Check sheet for the modelled part. Datum: model origin and axes. Units: mm. A direction names the side the tool comes from. Coordinates: 2 decimals unless noted, no trailing zeros. Loops run counter-clockwise (first coordinate to the right, second up) from the corner with the lowest first, then second, coordinate; pieces in that order, holes last. Notation, with made-up numbers: (15, -20.5) -> (37, -20.5) arc R16 ccw to (37, -12.5) -> close; hole circle Ø9 at (74.5, 29). An arc over 180 degrees is marked (long way). Use CSV: the item, a comma, the result in double quotes.
```python
from build123d import *

# Parameters (mm, degrees)
SKETCH_R           = 10.3
PAD_DEPTH          = 2
SKETCH001_R        = 4.3
SKETCH001_R_2      = 3.3
POCKET_DEPTH       = 1
SKETCH002_R        = 2.8
POCKET001_DEPTH    = 1
SKETCH003_R        = 1.5
POCKET002_DEPTH    = 1.001
SKETCH004_R        = 4.5
SKETCH004_R_2      = 3
PAD001_DEPTH       = 3
SKETCH005_R        = 0.75
POCKET003_DEPTH    = 5
POLARPATTERN_COUNT = 4


with BuildPart() as part:
    # Sketch → Pad (new body)
    with BuildSketch(Plane.XY):
        Circle(SKETCH_R)
    extrude(amount=PAD_DEPTH)

    # Sketch001 (on Face2 of Pad) → Pocket (cut)
    with BuildSketch(Plane(origin=(0, 0, 0), x_dir=(1, 0, 0), z_dir=(0, 0, -1))):
        Circle(SKETCH001_R)
        Circle(SKETCH001_R_2, mode=Mode.SUBTRACT)
    extrude(amount=-POCKET_DEPTH, mode=Mode.SUBTRACT)

    # Sketch002 (on Face7 of Pocket) → Pocket001 (cut)
    with BuildSketch(Plane(origin=(0, 0, 0), x_dir=(1, 0, 0), z_dir=(0, 0, -1))):
        Circle(SKETCH002_R)
    extrude(amount=-POCKET001_DEPTH, mode=Mode.SUBTRACT)

    # Sketch003 (on Face9 of Pocket001) → Pocket002 (cut, through all)
    with BuildSketch(Plane(origin=(0, 0, 1), x_dir=(1, 0, 0), z_dir=(0, 0, -1))):
        Circle(SKETCH003_R)
    extrude(amount=-POCKET002_DEPTH, mode=Mode.SUBTRACT)

    # Sketch004 (on Face3 of Pocket002) → Pad001 (join)
    with BuildSketch(Plane.XY.offset(2)):
        Circle(SKETCH004_R)
        Circle(SKETCH004_R_2, mode=Mode.SUBTRACT)
    extrude(amount=PAD001_DEPTH)

    # Sketch005 (on Face2 of Pad001) → Pocket003 (cut)
    with BuildSketch(Plane(origin=(0, 0, 0), x_dir=(1, 0, 0), z_dir=(0, 0, -1))):
        with Locations((-3.3, 7.3)):
            Circle(SKETCH005_R)
        with Locations((0, 7.3)):
            Circle(SKETCH005_R)
        with Locations((3.3, 7.3)):
            Circle(SKETCH005_R)
    pocket003 = extrude(amount=-POCKET003_DEPTH, mode=Mode.SUBTRACT)

    # PolarPattern: Pocket003 ×4 about axis
    polarpattern_axis = Axis((0, 0, 0), (0, 0, -1))
    for i in range(1, POLARPATTERN_COUNT):
        add(pocket003.rotate(polarpattern_axis, i * 360 / POLARPATTERN_COUNT), mode=Mode.SUBTRACT)


solid = part.part
```
1) Go/stop test with flat-tipped pins: pin 1 Ø2.5 at (x, y) = (0, 0) entering from -Z; pin 2 Ø2 at (x, y) = (3.3, 7.3) entering from -Z; pin 3 Ø1.7 at (x, y) = (7.3, -3.3) entering from +Z. Record where each tip stops, or that it passes through.
Answer below:
pin 1,"passes through"
pin 2,"stops at z = 0"
pin 3,"stops at z = 2"
2) Cross-section at A-A on x = -3.75. Record the boundary of the cut face in (y, z).
Answer below:
outline,"(-9.59, 0) -> (-7.9, 0) -> (-7.9, 2) -> (-9.59, 2) -> close; (-6.7, 0) -> (-2.1, 0) -> (-2.1, 1) -> (2.1, 1) -> (2.1, 0) -> (6.7, 0) -> (6.7, 2) -> (2.49, 2) -> (2.49, 5) -> (-2.49, 5) -> (-2.49, 2) -> (-6.7, 2) -> close; (7.9, 0) -> (9.59, 0) -> (9.59, 2) -> (7.9, 2) -> close"
3) Thickness scan on line 1 along Y through (x, z) = (0, 0.35); line 2 along Y through (x, z) = (0, 1.3); line 3 along Y through (x, z) = (0, 2.9). Record the ranges inside material, lowest first. Write a range as from..to.
Answer below:
line 1,"y = -10.3..-8.05, -6.55..-4.3, -3.3..-2.8, 2.8..3.3, 4.3..6.55, 8.05..10.3"
line 2,"y = -10.3..-8.05, -6.55..-1.5, 1.5..6.55, 8.05..10.3"
line 3,"y = -4.5..-3, 3..4.5"
4) Draft check along X on faces 4 (the cylindrical face through (9.824, 3.094, 0.986)), 5 (the flat face through (2.1, -4.4, 2)), 6 (the cylindrical face through (-3.202, 8.044, 0.986)), 7 (the cylindrical face through (-3, 0, 3)). Enter one of: released by +X, released by -X, zero draft, split by the parting line, or undercut.
Answer below:
face 4,"split by the parting line"
face 5,"zero draft"
face 6,"undercut"
face 7,"undercut"
5) Cross-section at B-B on x = 7.3. Record the boundary of the cut face in (y, z).
Answer below:
outline,"(-7.27, 0) -> (-4.05, 0) -> (-4.05, 2) -> (-7.27, 2) -> close; (-2.55, 0) -> (-0.75, 0) -> (-0.75, 2) -> (-2.55, 2) -> close; (0.75, 0) -> (2.55, 0) -> (2.55, 2) -> (0.75, 2) -> close; (4.05, 0) -> (7.27, 0) -> (7.27, 2) -> (4.05, 2) -> close"
6) Access from +Z, -Z, +X, -X, +Y, -Y to the whole of each face (thin tool, end or side, straight path). Record for faces 1 (the flat face through (1.3, -1.3, 2)), 2 (the flat face through (2, 3, 1)), 3 (the cylindrical face through (-8.044, 3.398, 0.986)).
Answer below:
face 1,"+Z"
face 2,"-Z"
face 3,"+Z, -Z"
7) Cross-section at C-C on y = 7. Record the boundary of the cut face in (x, z).
Answer below:
outline,"(-7.56, 0) -> (-3.99, 0) -> (-3.99, 2) -> (-7.56, 2) -> close; (-2.61, 0) -> (-0.69, 0) -> (-0.69, 2) -> (-2.61, 2) -> close; (0.69, 0) -> (2.61, 0) -> (2.61, 2) -> (0.69, 2) -> close; (3.99, 0) -> (7.56, 0) -> (7.56, 2) -> (3.99, 2) -> close"
8) Cross-section at D-D on z = 3.7. Record the boundary of the cut face in (x, y).
Answer below:
outline,"circle Ø9 at (0, 0); hole circle Ø6 at (0, 0)"
